Work out the finished part from the listing and answer in its coordinate system (mm). A direction names the side the tool comes from. Coordinates: 2 decimals unless noted, no trailing zeros. Write each loop counter-clockwise with the first axis right and the second up, starting at its lowest first coordinate (ties: lowest second). Pieces come first, ordered by that corner, then holes. Notation, with made-up numbers: M 28.5,-28 L 33.5,-28 A23 cw 33.5,10 Z; hole C -13,-38 d2. An arc over 180 degrees is marked long. Use CSV: the item, a comma, the result in double quotes.
from build123d import *

# Parameters (mm, degrees)
SKETCH_1_W                       = 64
SKETCH_1_H                       = 20
SM_BASE_FLANGE_1_DEPTH           = 1.5
SM_EDGE_FLANGE_1_STRIP_W         = 7.4732
SM_EDGE_FLANGE_1_STRIP_H         = 1.5
SM_EDGE_FLANGE_1_STRIP_CUT_DEPTH = 20
SM_EDGE_FLANGE_1_DEPTH           = 20
SM_EDGE_FLANGE_2_STRIP_W         = 7.4732
SM_EDGE_FLANGE_2_STRIP_H         = 1.5
SM_EDGE_FLANGE_2_STRIP_CUT_DEPTH = 20
SM_EDGE_FLANGE_2_DEPTH           = 20


# Sheet-metal steps are written as plain solids
with BuildPart() as part:
    # Sketch 1 → Базовая кромка1 (new body)
    with BuildSketch(Plane(origin=(0, 0, 0), x_dir=(1, 0, 0), z_dir=(0, 1, 0))):
        with Locations((32, 10)):
            Rectangle(SKETCH_1_W, SKETCH_1_H)
    extrude(amount=-SM_BASE_FLANGE_1_DEPTH)

    # Ребро-кромка1 strip (across the edge) → Ребро-кромка1 strip cut (cut)
    with BuildSketch(Plane.XY.offset(-20)):
        with Locations((-1.5, -0.75)):
            Rectangle(SM_EDGE_FLANGE_1_STRIP_W, SM_EDGE_FLANGE_1_STRIP_H)
    extrude(amount=SM_EDGE_FLANGE_1_STRIP_CUT_DEPTH, mode=Mode.SUBTRACT)

    # Ребро-кромка1 section (across the edge) → Ребро-кромка1 (add)
    with BuildSketch(Plane.XY.offset(-20)):
        with BuildLine():
            Line((0, 0.7366), (0, 35))
            Line((0, 35), (1.5, 35))
            Line((1.5, 35), (1.5, 0.7366))
            ThreePointArc((1.5, 0.7366), (1.715745145, 0.215745145), (2.2366, 0))
            Line((2.2366, 0), (2.2366, -1.5))
            ThreePointArc((2.2366, -1.5), (0.655084973, -0.844915027), (0, 0.7366))
        make_face()
    extrude(amount=SM_EDGE_FLANGE_1_DEPTH)

    # Ребро-кромка2 strip (across the edge) → Ребро-кромка2 strip cut (cut)
    with BuildSketch(Plane(origin=(64, 0, 0), x_dir=(-1, 0, 0), z_dir=(0, 0, -1))):
        with Locations((-1.5, -0.75)):
            Rectangle(SM_EDGE_FLANGE_2_STRIP_W, SM_EDGE_FLANGE_2_STRIP_H)
    extrude(amount=SM_EDGE_FLANGE_2_STRIP_CUT_DEPTH, mode=Mode.SUBTRACT)

    # Ребро-кромка2 section (across the edge) → Ребро-кромка2 (add)
    with BuildSketch(Plane(origin=(64, 0, 0), x_dir=(-1, 0, 0), z_dir=(0, 0, -1))):
        with BuildLine():
            Line((0, 0.7366), (0, 35))
            Line((0, 35), (1.5, 35))
            Line((1.5, 35), (1.5, 0.7366))
            ThreePointArc((1.5, 0.7366), (1.715745145, 0.215745145), (2.2366, 0))
            Line((2.2366, 0), (2.2366, -1.5))
            ThreePointArc((2.2366, -1.5), (0.655084973, -0.844915027), (0, 0.7366))
        make_face()
    extrude(amount=SM_EDGE_FLANGE_2_DEPTH)


solid = part.part
Item 1: The part is cut by section A-A (y = 5). Write down the section's boundary in (x, z).
Answer:
outline,"M 0,-20 L 1.5,-20 L 1.5,0 L 0,0 Z; M 62.5,-20 L 64,-20 L 64,0 L 62.5,0 Z"
Item 2: Given pin 1 (8 mm diameter, centred on x = 57, z = -10, fed in from +Y); pin 2 (10 mm diameter, centred on x = 44, y = 7.5, fed in from +Z), each flat-ended and moving along its own axis, determine where each tip first touches the part or whether it passes through.
Answer:
pin 1,"stops at y = 0"
pin 2,"passes through"
Item 3: A tool of negligible diameter and unlimited length cuts with its end or side. For faces 1 (the face through (1.5, 18, -10)), 2 (the face through (32, -1, -20)), from which of +Z, -Z, +X, -X, +Y, -Y can it reach the whole face along a straight path? Write none if from no direction.
Answer:
face 1,"+Z, -Z, +Y"
face 2,"-Z, +X, -X, +Y, -Y"
Item 4: The part is cut by section B-B (z = -3). Write down the section's boundary in (x, y), then the cut area to 3 significant figures.
Answer:
outline,"M 0,0.74 A2.24 ccw 2.24,-1.5 L 61.76,-1.5 A2.24 ccw 64,0.74 L 64,35 L 62.5,35 L 62.5,0.74 A0.74 cw 61.76,0 L 2.24,0 A0.74 cw 1.5,0.74 L 1.5,35 L 0,35 Z"
area,"199 mm2"
Item 5: Consider probe 1 along X at (y, z) = (18.5, -1.25); probe 2 along Y at (x, z) = (21, -16). Determine where each line is inside the solid, lowest interval first.
Answer:
probe 1,"x = 0 to 1.5, 62.5 to 64"
probe 2,"y = -1.5 to 0"
Item 6: The part is cut by section C-C (x = 5.5). Write down the section's boundary in (y, z), then the cut area to 3 significant figures.
Answer:
outline,"M -1.5,-20 L 0,-20 L 0,0 L -1.5,0 Z"
area,"30.0 mm2"
Item 7: For a pull along X with two mould halves and no side action, classify faces 3 (the face through (32, 0, -10)), 4 (the face through (63.33, -0.86, -9.86)), 5 (the face through (63, 35, -10)), 6 (the face through (0, 18, -10)) as released by +X, released by -X, zero draft, split by the parting line, or undercut.
Answer:
face 3,"undercut"
face 4,"released by +X"
face 5,"zero draft"
face 6,"released by -X"
